```python
from build123d import *

# Parameters (mm, degrees)
BOSS_EXTRUDE1_DEPTH = 63.5
SKETCH7_R           = 44.704
CUT_EXTRUDE1_DEPTH  = 50.8
SKETCH8_R           = 3.302
CUT_EXTRUDE2_DEPTH  = 18.526
SKETCH9_R           = 5.588
CUT_EXTRUDE3_DEPTH  = 10.144


with BuildPart() as part:
    # Sketch2 → Boss-Extrude1 (new body)
    with BuildSketch(Plane.XY):
        with BuildLine():
            Line((-33.02, 0), (-33.02, 7.366))
            ThreePointArc((-33.02, 7.366), (-28.240847698, 15.984124973), (-18.399512195, 16.494507465))
            ThreePointArc((-18.399512195, 16.494507465), (0, 12.239600759), (18.399512195, 16.494507465))
            ThreePointArc((18.399512195, 16.494507465), (28.240847698, 15.984124973), (33.02, 7.366))
            Line((33.02, 7.366), (33.02, 0))
            Line((33.02, 0), (-33.02, 0))
        make_face()
    extrude(amount=-BOSS_EXTRUDE1_DEPTH)

    # Sketch7 → Cut-Extrude1 (cut)
    with BuildSketch(Plane.XY):
        with Locations((0, 54.149600759)):
            Circle(SKETCH7_R)
    extrude(amount=-CUT_EXTRUDE1_DEPTH, mode=Mode.SUBTRACT)

    # Sketch8 → Cut-Extrude2 (cut, through all)
    with BuildSketch(Plane(origin=(0, 0, 0), x_dir=(-1, 0, 0), z_dir=(0, -1, 0))):
        with Locations((19.05, 19.05)):
            Circle(SKETCH8_R)
        with Locations((-19.05, 19.05)):
            Circle(SKETCH8_R)
    extrude(amount=-CUT_EXTRUDE2_DEPTH, mode=Mode.SUBTRACT)

    # Sketch9 → Cut-Extrude3 (cut, through all)
    with BuildSketch(Plane(origin=(0, 8.382, 0), x_dir=(-1, 0, 0), z_dir=(0, -1, 0))):
        with Locations((19.05, 19.05)):
            Circle(SKETCH9_R)
        with Locations((-19.05, 19.05)):
            Circle(SKETCH9_R)
    extrude(amount=-CUT_EXTRUDE3_DEPTH, mode=Mode.SUBTRACT)


solid = part.part
```
Design review of the part built by this model. Coordinates are the model's own, in mm. A direction names the side the tool comes from. Give positions to 0.01 mm unless a question says otherwise; leave off trailing zeros. Write each loop counter-clockwise with the first axis right and the second up, starting at its lowest first coordinate (ties: lowest second). Pieces come first, ordered by that corner, then holes. Notation, with made-up numbers: (35, -10) - (58, -10) arc R13 cw to (58, -1) - close; hole circle Ø6 at (73, 22.5). An arc over 180 degrees is marked (long way). Return JSON: item names as keys, results as strings. Group by question number.
(1) Machinability: for faces 1 (the flat face through (33.02, 4, -31)), 2 (the cylindrical face through (-0.375, 9.447, -25.044)), 3 (the cylindrical face through (-24.38, 11.62, -20.73)), which of the approach directions +Z, -Z, +X, -X, +Y, -Y give a long, thin tool a straight path to every point of the face, cutting with its end or side? Answer none if there is none.
(2) We need section C-C, the plane z = -19.05. Give the boundary of the cut face in (x, y).
(3) We need section A-A, the plane z = -11.5. Give the boundary of the cut face in (x, y).
(4) Insertion check: pin 1 (1.5 mm diameter, centred on x = -13.5, y = 15, fed in from +Z); pin 2 (6 mm diameter, centred on x = 1.5, z = -17.5, fed in from +Y); pin 3 (2 mm diameter, centred on x = 11.5, z = -24.5, fed in from +Y). Each pin has a flat end and moves straight along its axis. Give the tip position at first contact, or say it passes through.
(5) Mouldability with a two-part tool opening along X and no side actions: class faces 4 (the flat face through (16.6, 8.382, -16.6)), 5 (the flat face through (0, 7, -63.5)), 6 (the flat face through (-33.02, 4, -31)) as +X half, -X half, draft (parallel to the pull), parting line (faces both ways), or undercut.
(6) To check wall thickness, follow probe 1 along Z at (x, y) = (19.05, 12); probe 2 along X at (y, z) = (4.75, -19.5); probe 3 along X at (y, z) = (15.75, -41.5). State the ranges of each line that lie inside material, in increasing order.
(7) We need section B-B, the plane x = -3. Give the boundary of the cut face in (y, z), then the cut area to 3 significant figures.
Reported:
{
 "1": {"face 1": "+Z, -Z, +X, +Y, -Y", "face 2": "+Z, +Y", "face 3": "+Y"},
 "2": {"outline": "(-33.02, 0) - (-22.35, 0) - (-22.35, 8.38) - (-24.64, 8.38) - (-24.64, 16.85) arc R44.7 cw to (-25.23, 17.25) arc R10.16 ccw to (-33.02, 7.37) - close; (-15.75, 0) - (15.75, 0) - (15.75, 8.38) - (13.46, 8.38) - (13.46, 11.52) arc R44.7 cw to (-13.46, 11.52) - (-13.46, 8.38) - (-15.75, 8.38) - close; (22.35, 0) - (33.02, 0) - (33.02, 7.37) arc R10.16 ccw to (25.23, 17.25) arc R44.7 cw to (24.64, 16.85) - (24.64, 8.38) - (22.35, 8.38) - close"},
 "3": {"outline": "(-33.02, 0) - (33.02, 0) - (33.02, 7.37) arc R10.16 ccw to (25.23, 17.25) arc R44.7 cw to (-25.23, 17.25) arc R10.16 ccw to (-33.02, 7.37) - close"},
 "4": {"pin 1": "stops at z = -50.8", "pin 2": "stops at y = 9.67", "pin 3": "stops at y = 11.23"},
 "5": {"face 4": "undercut", "face 5": "draft", "face 6": "-X half"},
 "6": {"probe 1": "z = -63.5 to -24.64, -13.46 to 0", "probe 2": "x = -33.02 to -22.32, -15.78 to 15.78, 22.32 to 33.02", "probe 3": "x = -28.6 to -22.89, 22.89 to 28.6"},
 "7": {"outline": "(0, -63.5) - (12.35, -63.5) - (12.35, -50.8) - (9.55, -50.8) - (9.55, 0) - (0, 0) - close", "area": "642 mm2"}
}
